from build123d import *

# Parameters (mm, degrees)
SKETCH_1_R      = 5
SKETCH_1_R_2    = 2.5
EXTRUDE_1_DEPTH = 8
SKETCH_2_R      = 11
SKETCH_2_R_2    = 2.5
SKETCH_2_R_3    = 1.6
EXTRUDE_2_DEPTH = 2.5


with BuildPart() as part:
    # 草图1 → 凸台-拉伸1 (new body)
    with BuildSketch(Plane(origin=(0, 0, 0), x_dir=(1, 0, 0), z_dir=(0, 1, 0))):
        with Locations(Location((0, 0, 0), (0, 0, 270))):
            Circle(SKETCH_1_R)
        with Locations(Location((0, 0, 0), (0, 0, 270))):
            Circle(SKETCH_1_R_2, mode=Mode.SUBTRACT)
    extrude(amount=EXTRUDE_1_DEPTH)

    # 草图2 → 凸台-拉伸2 (add)
    with BuildSketch(Plane(origin=(0, 8, 0), x_dir=(-1, 0, 0), z_dir=(0, 1, 0))):
        with Locations(Location((0, 0, 0), (0, 0, 90))):
            Circle(SKETCH_2_R)
        with Locations(Location((0, 0, 0), (0, 0, 90))):
            Circle(SKETCH_2_R_2, mode=Mode.SUBTRACT)
        with Locations(Location((-8, 0, 0), (0, 0, 90))):
            Circle(SKETCH_2_R_3, mode=Mode.SUBTRACT)
        with Locations(Location((0, 8, 0), (0, 0, 90))):
            Circle(SKETCH_2_R_3, mode=Mode.SUBTRACT)
        with Locations(Location((8, 0, 0), (0, 0, 90))):
            Circle(SKETCH_2_R_3, mode=Mode.SUBTRACT)
        with Locations(Location((0, -8, 0), (0, 0, 90))):
            Circle(SKETCH_2_R_3, mode=Mode.SUBTRACT)
    extrude(amount=EXTRUDE_2_DEPTH)


solid = part.part
Source: CAD feature listing. Evaluate the final solid. Frame: model axes, mm. A direction names the side the tool comes from. Round coordinates to 2 decimals unless told otherwise and drop trailing zeros. Loops run counter-clockwise (first coordinate to the right, second up) from the corner with the lowest first, then second, coordinate; pieces in that order, holes last. Notation, with made-up numbers: (17, 74) -> (35, 74) arc R26 ccw to (35, 110) -> close; hole circle Ø2 at (80, -28.5). An arc over 180 degrees is marked (long way). Answer as a JSON object with one key per item and string values. Group by question number.
Q1. Section query C-C (x = -8). Output: boundary loops of the cut face in (y, z), plus the area to 3 significant figures.
Q2. Section query D-D (z = -8). Output: boundary loops of the cut face in (x, y), plus the area to 3 significant figures.
Q3. Section query A-A (z = 0). Output: boundary loops of the cut face in (x, y), plus the area to 3 significant figures.
Q4. Contact query for flat-ended pins moving along their axis: P1, Ø6, axis at x = -8, z = -4.5, coming from the -Y side; P2, Ø1.9, axis at x = 0, z = 8, coming from the +Y side; P3, Ø2, axis at x = -5, y = 3.5, coming from the +Z side; P4, Ø5, axis at y = 7, z = 4.5, coming from the +X side. Output: stop coordinate, or through.
Q5. Access query for faces 1 (the cylindrical face through (-4.88, 3.94, -1.08)), 2 (the cylindrical face through (0.07, 9.23, -9.6)). Directions: +Z, -Z, +X, -X, +Y, -Y. A direction counts if a zero-diameter tool reaches every point of the face in a straight line with its end or side. Return the directions, or none.
Q6. Mould query, pull axis X, two halves, no side actions, for faces 3 (the flat face through (-2, 0, 2)), 4 (the cylindrical face through (0.07, 9.23, 6.4)), 5 (the cylindrical face through (-10.74, 9.23, -2.38)). Classes: pulls with the +X half, pulls with the -X half, needs draft (parallel to the pull), parting line crosses it, or undercut.
Q7. Section query B-B (x = -1.25). Output: boundary loops of the cut face in (y, z), plus the area to 3 significant figures.
Q8. Ray query, line 1 (X direction, y = 9.5, z = 0); line 2 (X direction, y = 6.75, z = 0); line 3 (X direction, y = 5.25, z = -1.25). Return the intervals inside material, ascending. Write a range as from..to.
Completed:
{
 "1": {"outline": "(8, -7.55) -> (10.5, -7.55) -> (10.5, -1.6) -> (8, -1.6) -> close; (8, 1.6) -> (10.5, 1.6) -> (10.5, 7.55) -> (8, 7.55) -> close", "area": "29.7 mm²"},
 "2": {"outline": "(-7.55, 8) -> (-1.6, 8) -> (-1.6, 10.5) -> (-7.55, 10.5) -> close; (1.6, 8) -> (7.55, 8) -> (7.55, 10.5) -> (1.6, 10.5) -> close", "area": "29.7 mm²"},
 "3": {"outline": "(-11, 8) -> (-9.6, 8) -> (-9.6, 10.5) -> (-11, 10.5) -> close; (-6.4, 8) -> (-5, 8) -> (-5, 0) -> (-2.5, 0) -> (-2.5, 10.5) -> (-6.4, 10.5) -> close; (2.5, 0) -> (5, 0) -> (5, 8) -> (6.4, 8) -> (6.4, 10.5) -> (2.5, 10.5) -> close; (9.6, 8) -> (11, 8) -> (11, 10.5) -> (9.6, 10.5) -> close", "area": "66.5 mm²"},
 "4": {"P1": "y = 8", "P2": "through", "P3": "z = 3", "P4": "x = 10.78"},
 "5": {"face 1": "-Y", "face 2": "+Y, -Y"},
 "6": {"face 3": "needs draft", "face 4": "undercut", "face 5": "parting line crosses it"},
 "7": {"outline": "(0, -4.84) -> (8, -4.84) -> (8, -7) -> (10.5, -7) -> (10.5, -2.17) -> (0, -2.17) -> close; (0, 2.17) -> (10.5, 2.17) -> (10.5, 7) -> (8, 7) -> (8, 4.84) -> (0, 4.84) -> close; (8, -10.93) -> (10.5, -10.93) -> (10.5, -9) -> (8, -9) -> close; (8, 9) -> (10.5, 9) -> (10.5, 10.93) -> (8, 10.93) -> close", "area": "76.6 mm²"},
 "8": {"line 1": "-11..-9.6, -6.4..-2.5, 2.5..6.4, 9.6..11", "line 2": "-5..-2.5, 2.5..5", "line 3": "-4.84..-2.17, 2.17..4.84"}
}
